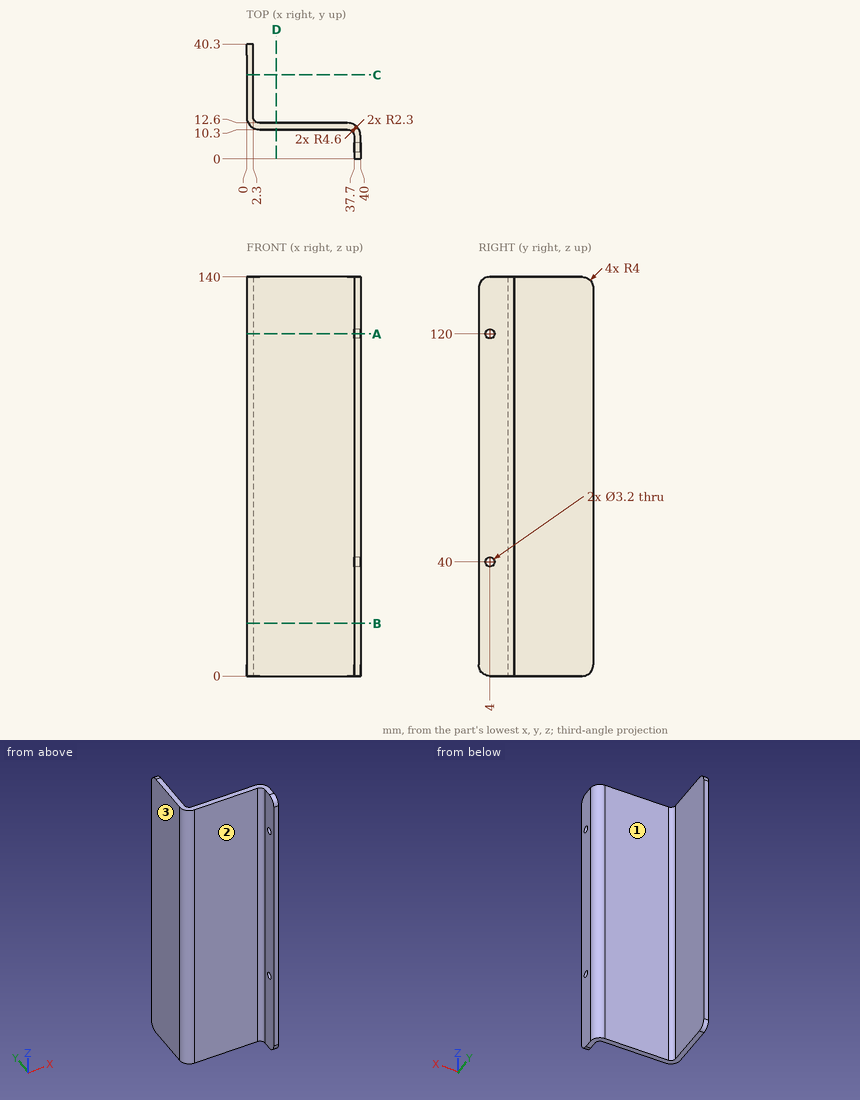
Job drawing, mm, ordinate dimensions from the low corner. One solid piece. A direction names the side the tool comes from. Round coordinates to 2 decimals unless told otherwise and drop trailing zeros. Loops run counter-clockwise (first coordinate to the right, second up) from the corner with the lowest first, then second, coordinate; pieces in that order, holes last. Notation, with made-up numbers: (83.25, -2) -> (142.25, -2) arc R21 ccw to (142.25, 24) -> close; hole circle Ø5 at (-3.75, 23). An arc over 180 degrees is marked (long way). Use a Markdown table: item, result.
1) Cut at A-A, the plane z = 120. List the corners of the cut face in (x, y), and give its area (3 significant figures).
The answers:
| item | result |
|---|---|
| outline | (0, 14.9) arc R4.6 ccw to (4.6, 10.3) -> (35.4, 10.3) arc R2.3 cw to (37.7, 8) -> (37.7, 5.6) -> (40, 5.6) -> (40, 8) arc R4.6 ccw to (35.4, 12.6) -> (4.6, 12.6) arc R2.3 cw to (2.3, 14.9) -> (2.3, 40.3) -> (0, 40.3) -> close; (37.7, 0) -> (40, 0) -> (40, 2.4) -> (37.7, 2.4) -> close |
| area | 165 mm2 |
2) Cut at B-B, the plane z = 18.5. List the corners of the cut face in (x, y), and give its area (3 significant figures).
The answers:
| item | result |
|---|---|
| outline | (0, 14.9) arc R4.6 ccw to (4.6, 10.3) -> (35.4, 10.3) arc R2.3 cw to (37.7, 8) -> (37.7, 0) -> (40, 0) -> (40, 8) arc R4.6 ccw to (35.4, 12.6) -> (4.6, 12.6) arc R2.3 cw to (2.3, 14.9) -> (2.3, 40.3) -> (0, 40.3) -> close |
| area | 173 mm2 |
3) Cut at D-D, the plane x = 10.5. List the corners of the cut face in (y, z).
The answers:
| item | result |
|---|---|
| outline | (10.3, 0) -> (12.6, 0) -> (12.6, 140) -> (10.3, 140) -> close |
4) Cut at C-C, the plane y = 29.5. List the corners of the cut face in (x, z).
The answers:
| item | result |
|---|---|
| outline | (0, 0) -> (2.3, 0) -> (2.3, 140) -> (0, 140) -> close |
5) Probe line 1 (X direction, y = 17, z = 8); line 2 (Y direction, x = 8, z = 104); line 3 (Y direction, x = 39, z = 40). List the from-to ranges inside material, lowest first. Write a range as [from, to].
The answers:
| item | result |
|---|---|
| line 1 | x = [0, 2.3] |
| line 2 | y = [10.3, 12.6] |
| line 3 | y = [0, 2.4], [5.6, 10.86] |
6) Drop flat-ended pins along their axis: pin 1 Ø20.5 at (y, z) = (24, 99) entering from +X; pin 2 Ø4 at (x, z) = (6, 120.5) entering from +Y; pin 3 Ø5 at (y, z) = (17, 87) entering from +X. Give the stop position or say it passes through.
The answers:
| item | result |
|---|---|
| pin 1 | stops at x = 2.61 |
| pin 2 | stops at y = 12.68 |
| pin 3 | stops at x = 2.34 |
7) Tool access for the marked faces 1, 2 and 3: list every direction of +Z, -Z, +X, -X, +Y, -Y with a clear straight run to the whole face (end or side of a thin tool).
The answers:
| item | result |
|---|---|
| face 1 | +Z, -Z, +X, +Y |
| face 2 | +Z, -Z, -X, -Y |
| face 3 | +Z, -Z, -X, +Y, -Y |
